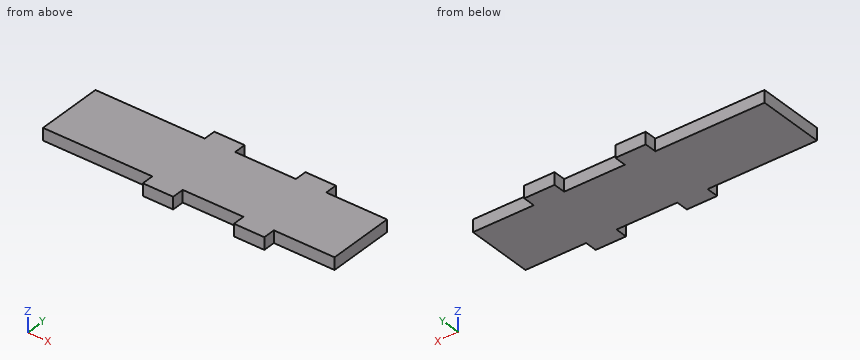
Autodesk Inventor part; units mm, degrees
ref_plane "YZ Plane" through (0, 0, 0) normal (1, 0, 0) x (0, 1, 0)
ref_plane "XZ Plane" through (0, 0, 0) normal (0, 1, 0) x (-1, 0, 0)
ref_plane "XY Plane" through (0, 0, 0) normal (0, 0, 1) x (1, 0, 0)
sketch "Sketch1" plane through (0, 0, 0) normal (0, 0, 1) x (1, 0, 0)
  line L0 (0, 4) -> (0, 26)
  line L1 (0, 26) -> (36, 26)
  line L2 (36, 26) -> (36, 30)
  line L3 (36, 30) -> (46, 30)
  line L4 (46, 30) -> (46, 26)
  line L5 (46, 26) -> (66, 26)
  line L6 (66, 26) -> (66, 30)
  line L7 (66, 30) -> (76, 30)
  line L8 (76, 30) -> (76, 26)
  line L9 (76, 26) -> (96, 26)
  line L10 (96, 26) -> (96, 4)
  line L11 (96, 4) -> (76, 4)
  line L12 (76, 4) -> (76, 0)
  line L13 (76, 0) -> (66, 0)
  line L14 (66, 0) -> (66, 4)
  line L15 (66, 4) -> (46, 4)
  line L16 (46, 4) -> (46, 0)
  line L17 (46, 0) -> (36, 0)
  line L18 (36, 4) -> (0, 4)
  line L19 (36, 0) -> (36, 4)
  point P0 (0, 0)
  dimension "d0" = 22
  dimension "d1" = 36
  dimension "d2" = 4
  dimension "d3" = 10
  dimension "d4" = 20
  dimension "d5" = 10
  dimension "d6" = 20
extrude "Extrusion1" add sketch "Sketch1" along normal blind 4
properties part number "hlid"
Work out the finished part from the listing and answer in its coordinate system (mm). Give positions to 0.01 mm unless a question says otherwise; leave off trailing zeros. Loops run counter-clockwise (first coordinate to the right, second up) from the corner with the lowest first, then second, coordinate; pieces in that order, holes last. Notation, with made-up numbers: (56, -36.75) - (78, -36.75) arc R16 ccw to (78, -6.75) - close; hole circle Ø3 at (81, -32.5). An arc over 180 degrees is marked (long way). Answer in a Markdown table with one row per item. Add a question column.
Q1. The part is cut by section B-B (z = 1.95). Determine the outline of the cut face in (x, y), and give its area (3 significant figures).
Q2. The part is cut by section A-A (y = 3). Determine the outline of the cut face in (x, z), and give its area (3 significant figures).
Q3. The part is cut by section C-C (x = 86). Determine the outline of the cut face in (y, z), and give its area (3 significant figures).
Q4. Each of these flat-tipped pins is pushed along its axis until it touches: P1, Ø1.2, axis at y = 29, z = 2, coming from the +X side; P2, Ø1.2, axis at x = 26.5, z = 1, coming from the -Y side; P3, Ø1.2, axis at x = 19, z = 1, coming from the +Y side. Where does it stop, or does it pass through?
Q5. Consider line 1 along X through (y, z) = (2, 0.65); line 2 along Y through (x, z) = (87.5, 1.45). Determine where each line is inside the solid, lowest interval first.
Solution:
| question | item | result |
|---|---|---|
| 1 | outline | (0, 4) - (36, 4) - (36, 0) - (46, 0) - (46, 4) - (66, 4) - (66, 0) - (76, 0) - (76, 4) - (96, 4) - (96, 26) - (76, 26) - (76, 30) - (66, 30) - (66, 26) - (46, 26) - (46, 30) - (36, 30) - (36, 26) - (0, 26) - close |
| 1 | area | 2,270 mm² |
| 2 | outline | (36, 0) - (46, 0) - (46, 4) - (36, 4) - close; (66, 0) - (76, 0) - (76, 4) - (66, 4) - close |
| 2 | area | 80.0 mm² |
| 3 | outline | (4, 0) - (26, 0) - (26, 4) - (4, 4) - close |
| 3 | area | 88.0 mm² |
| 4 | P1 | stops at x = 76 |
| 4 | P2 | stops at y = 4 |
| 4 | P3 | stops at y = 26 |
| 5 | line 1 | x = 36 to 46, 66 to 76 |
| 5 | line 2 | y = 4 to 26 |
